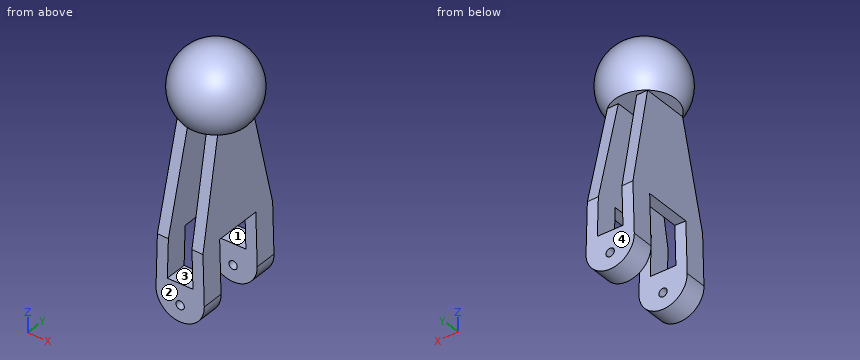
```python
from build123d import *

# Parameters (mm, degrees)
BOSS_EXTRUDE1_DEPTH     = 53.34
SKETCH4_W               = 61.072672184
SKETCH4_H               = 27.686
CUT_EXTRUDE3_DEPTH      = 29.259495037
SKETCH5_OUTSIDE_W       = 57.352
SKETCH5_OUTSIDE_H       = 152.814
CUT_EXTRUDE5_DEPTH      = 54.34
SKETCH6_R               = 2.413
CUT_EXTRUDE6_DEPTH      = 54.34
CUT_EXTRUDE8_DEPTH      = 100
CUT_EXTRUDE8_DEPTH_BACK = 100
CUT_EXTRUDE9_DEPTH      = 100


with BuildPart() as part:
    # Sketch1 → Boss-Extrude1 (new body)
    with BuildSketch(Plane(origin=(0, 0, 0), x_dir=(1, 0, 0), z_dir=(0, 1, 0))):
        with BuildLine():
            Line((-13.944778991, -0.365156889), (-11.616850564, -89.265156889))
            ThreePointArc((-11.616850564, -89.265156889), (0, -109.412099434), (11.616850564, -89.265156889))
            Line((11.616850564, -89.265156889), (13.944778991, -0.365156889))
            ThreePointArc((13.944778991, -0.365156889), (0, 13.949559157), (-13.944778991, -0.365156889))
        make_face()
    extrude(amount=BOSS_EXTRUDE1_DEPTH)

    # Sketch4 → Cut-Extrude3 (cut, through all)
    with BuildSketch(Plane(origin=(13.944778991, 0, 0.365156889), x_dir=(0.026176948, 0, -0.999657325), z_dir=(0.999657325, 0, 0.026176948))):
        with Locations((0, 26.67)):
            Rectangle(SKETCH4_W, SKETCH4_H)
    extrude(amount=-CUT_EXTRUDE3_DEPTH, mode=Mode.SUBTRACT)

    # Sketch5 outside → Cut-Extrude5 (cut, through all)
    with BuildSketch(Plane(origin=(0, 53.34, 0), x_dir=(1, 0, 0), z_dir=(0, 1, 0))):
        with Locations((0, -47.731)):
            Rectangle(SKETCH5_OUTSIDE_W, SKETCH5_OUTSIDE_H)
        with BuildLine():
            Line((-13.944778991, -0.365156889), (-11.616850564, -89.265156889))
            ThreePointArc((-11.616850564, -89.265156889), (0, -109.412099434), (11.616850564, -89.265156889))
            Line((11.616850564, -89.265156889), (13.944778991, -0.365156889))
            ThreePointArc((13.944778991, -0.365156889), (0, 13.949559157), (-13.944778991, -0.365156889))
        make_face(mode=Mode.SUBTRACT)
        with BuildLine():
            Line((7.403977553, -7.568443783), (5.213735587, -91.210409969))
            ThreePointArc((5.213735587, -91.210409969), (0, -105.33899845), (-5.213735587, -91.210409969))
            Line((-5.213735587, -91.210409969), (-7.403977553, -7.568443783))
            Line((-7.403977553, -7.568443783), (7.403977553, -7.568443783))
        make_face()
    extrude(amount=-CUT_EXTRUDE5_DEPTH, mode=Mode.SUBTRACT)

    # Sketch6 → Cut-Extrude6 (cut, through all)
    with BuildSketch(Plane(origin=(0, 53.34, 0), x_dir=(1, 0, 0), z_dir=(0, 1, 0))):
        with Locations((0, 4.57874024)):
            Circle(SKETCH6_R)
    extrude(amount=-CUT_EXTRUDE6_DEPTH, mode=Mode.SUBTRACT)

    # Sketch7 → Cut-Extrude8 (cut, two sides)
    with BuildSketch(Plane(origin=(-13.944778991, 0, 0.365156889), x_dir=(0.026176948, 0, 0.999657325), z_dir=(-0.999657325, 0, 0.026176948))) as cut_extrude8_sk:
        Polygon((29.847177093, 53.34), (88.930474252, 40.09), (115.196693912, 40.09), (115.196693912, 13.25), (88.930474252, 13.25), (29.847177093, 0), (138.702727396, 0), (138.702727396, 53.34), align=None)
    extrude(amount=CUT_EXTRUDE8_DEPTH, mode=Mode.SUBTRACT)
    extrude(cut_extrude8_sk.sketch, amount=-CUT_EXTRUDE8_DEPTH_BACK, mode=Mode.SUBTRACT)

    # Sketch8 → Cut-Extrude9 (cut)
    with BuildSketch(Plane(origin=(0, 40.09, 0), x_dir=(1, 0, 0), z_dir=(0, 1, 0))):
        Polygon((-11.616850564, -89.265156889), (19.748470708, -88.443827046), (21.136276119, -119.73242467), (-27.769338844, -116.21935592), (-20.465853811, -89.265156889), align=None)
    extrude(amount=-CUT_EXTRUDE9_DEPTH, mode=Mode.SUBTRACT)

    # Sketch14 one side → Revolve6 (revolve)
    with BuildSketch(Plane(origin=(0, 26.771336555, 0), x_dir=(-0.999657325, 0, 0.026176948), z_dir=(0, 1, 0))):
        with BuildLine():
            Line((-15.398394592, 88.930474252), (-9.308054112, 88.930474252))
            Line((-9.308054112, 88.930474252), (2.320752522, 88.930474252))
            Line((2.320752522, 88.930474252), (2.320752522, 103.921360067))
            Line((2.320752522, 103.921360067), (2.320752522, 127.13116041))
            ThreePointArc((2.320752522, 127.13116041), (-18.734297925, 113.687612297), (-15.398394592, 88.930474252))
        make_face()
    revolve(axis=Axis((0.400386812, 26.771336555, 103.946499032), (0.026176948, 0, 0.999657325)))


solid = part.part
```
Work out the finished part from the listing and answer in its coordinate system (mm). Face numbers are marked on the shaded views. A direction names the side the tool comes from. Round coordinates to 2 decimals unless told otherwise and drop trailing zeros. Order: outer loops, then holes, each group sorted by start corner. A loop starts at its lowest first (then second) coordinate and runs counter-clockwise, first axis right, second up.
Q1. The mould has two halves that part along Z. Classify the marked faces 3 and 4: pulls with the +Z half, pulls with the -Z half, needs draft (parallel to the pull), parting line crosses it, or undercut.
Solution:
face 3: undercut
face 4: needs draft
Q2. A cutting plane is placed at B-B, the plane y = 48.5. Determine the outline of the cut face in (x, z), then the cut area to 3 significant figures.
Solution:
outline: (-13.94, 0.37) arc R13.95 ccw (long way) to (13.94, 0.37) - (12.62, 51.12) - (6.26, 51.28) - (7.4, 7.57) - (-7.4, 7.57) - (-6.25, 51.61) - (-12.6, 51.78) - close; circle Ø16.32 at (0.4, 103.95); hole circle Ø4.83 at (0, -4.58)
area: 1,260 mm2
Q3. A cutting plane is placed at C-C, the plane y = 33. Determine the outline of the cut face in (x, z), then the cut area to 3 significant figures.
Solution:
outline: (-16.57, 89.39) - (-11.62, 89.27) - (-13.16, 30.2) - (-6.81, 30.37) - (-5.27, 89.1) - (5.28, 88.82) - (6.8, 30.72) - (13.15, 30.89) - (11.63, 88.66) - (16.59, 88.53) arc R22.36 ccw (long way) to start
area: 2,140 mm2
Q4. Given pin 1 Ø4 at (x, y) = (-1, 8) entering from +Z; pin 2 Ø2 at (x, y) = (3.5, 14) entering from -Z; pin 3 Ø14 at (x, y) = (-3, 48) entering from +Z, each flat-ended and moving along its own axis, determine where each tip first touches the part or whether it passes through.
Solution:
pin 1: stops at z = 119.94
pin 2: stops at z = 88.84
pin 3: stops at z = 122.07
Q5. Find the intervals of material crossed by line 1 along Y through (x, z) = (-13, 16.5); line 2 along Z through (x, y) = (0, 50.75); line 3 along Z through (x, y) = (0, 6.5), in increasing order.
Solution:
line 1: y = 0 to 12.83, 40.51 to 53.34
line 2: z = -13.95 to -6.99, -2.17 to 7.57
line 3: z = -13.95 to -6.99, -2.17 to 7.57, 92.65 to 115.24
Q6. A cutting plane is placed at A-A, the plane z = 71. Determine the outline of the cut face in (x, y).
Solution:
outline: (-12.1, 9.15) - (-5.74, 9.19) - (-5.74, 44.15) - (-12.1, 44.19) - close; (5.74, 9.26) - (12.1, 9.29) - (12.1, 44.05) - (5.74, 44.08) - close
Q7. A tool of negligible diameter and unlimited length cuts with its end or side. For the marked faces 1 and 2, from which of +Z, -Z, +X, -X, +Y, -Y can it reach the whole face along a straight path? Write none if from no direction.
Solution:
face 1: +Y, -Y
face 2: +Z, -Z, +X, -X, -Y
Q8. A cutting plane is placed at D-D, the plane z = 53. Determine the outline of the cut face in (x, y).
Solution:
outline: (-12.57, 5.11) - (-6.21, 5.15) - (-6.21, 48.19) - (-12.57, 48.23) - close; (6.21, 5.22) - (12.57, 5.26) - (12.57, 48.08) - (6.21, 48.12) - close
